```python
from build123d import *

# Parameters (mm, degrees)
SKETCH_W     = 53
SKETCH_H     = 50
PAD_DEPTH    = 2
SKETCH001_R  = 1.6
PAD001_DEPTH = 2
SKETCH002_R  = 1.6
PAD002_DEPTH = 2
SKETCH003_W  = 53
SKETCH003_H  = 4
PAD003_DEPTH = 6
POCKET_DEPTH = 50
FILLET_R     = 5


with BuildPart() as part:
    # Sketch → Pad (new body)
    with BuildSketch(Plane.YZ.offset(27)):
        Rectangle(SKETCH_W, SKETCH_H)
    extrude(amount=PAD_DEPTH)

    # Sketch001 (on Face4 of Pad) → Pad001 (join)
    with BuildSketch(Plane(origin=(27, -26.5, 0), x_dir=(0, 0, -1), z_dir=(0, -1, 0))):
        with BuildLine():
            Line((-32.5, 2), (32.5, 2))
            ThreePointArc((32.5, -8), (37.5, -3), (32.5, 2))
            Line((-32.5, -8), (32.5, -8))
            ThreePointArc((-32.5, 2), (-37.5, -3), (-32.5, -8))
        make_face()
        with Locations((-32.5, -3)):
            Circle(SKETCH001_R, mode=Mode.SUBTRACT)
        with Locations((32.5, -3)):
            Circle(SKETCH001_R, mode=Mode.SUBTRACT)
    extrude(amount=PAD001_DEPTH)

    # Sketch002 (on Face13 of Pad001) → Pad002 (join)
    with BuildSketch(Plane(origin=(27, 26.5, 0), x_dir=(0, 0, 1), z_dir=(0, 1, 0))):
        with BuildLine():
            Line((-32.5, 2), (32.5, 2))
            ThreePointArc((32.5, -8), (37.5, -3), (32.5, 2))
            Line((32.5, -8), (-32.5, -8))
            ThreePointArc((-32.5, 2), (-37.5, -3), (-32.5, -8))
        make_face()
        with Locations((-32.5, -3)):
            Circle(SKETCH002_R, mode=Mode.SUBTRACT)
        with Locations((32.5, -3)):
            Circle(SKETCH002_R, mode=Mode.SUBTRACT)
    extrude(amount=PAD002_DEPTH)

    # Sketch003 (on Face8 of Pad002) → Pad003 (join)
    with BuildSketch(Plane(origin=(27, 0, 0), x_dir=(0, 1, 0), z_dir=(-1, 0, 0))):
        with Locations((0, -15)):
            Rectangle(SKETCH003_W, SKETCH003_H)
        with Locations((0, 15)):
            Rectangle(SKETCH003_W, SKETCH003_H)
    extrude(amount=PAD003_DEPTH)

    # Sketch004 (on Face9 of Pad003) → Pocket (cut)
    with BuildSketch(Plane(origin=(27, 0, -17), x_dir=(0, 1, 0), z_dir=(0, 0, -1))):
        with BuildLine():
            ThreePointArc((-7, 0), (-7.942809, -0.390524), (-8.333333, -1.333333))
            Line((-8.333333, -2.666667), (-8.333333, -1.333333))
            ThreePointArc((-8.333333, -2.666667), (-7.942809, -3.609476), (-7, -4))
            Line((7, -4), (-7, -4))
            ThreePointArc((7, -4), (7.942809, -3.609476), (8.333333, -2.666667))
            Line((8.333333, -1.333333), (8.333333, -2.666667))
            ThreePointArc((8.333333, -1.333333), (7.942809, -0.390524), (7, 0))
            Line((-7, 0), (7, 0))
        make_face()
    extrude(amount=-POCKET_DEPTH, mode=Mode.SUBTRACT)

    # Fillet
    fillet_edges = [part.edges().sort_by_distance(p)[0] for p in [
        (27, 26.5, 0),
        (27, -26.5, 0),
        (27, 26.5, 21),
        (27, -26.5, 21),
        (27, -26.5, -21),
        (27, 26.5, -21),
    ]]
    fillet(fillet_edges, radius=FILLET_R)


solid = part.part
```
Design review of the part built by this model. Coordinates are the model's own, in mm. A direction names the side the tool comes from. Round coordinates to 2 decimals unless told otherwise and drop trailing zeros. Write each loop counter-clockwise with the first axis right and the second up, starting at its lowest first coordinate (ties: lowest second). Pieces come first, ordered by that corner, then holes.
Item 1: For faces 4 (the flat face through (21, 0, 15)), 5 (the cylindrical face through (25.57, -25, 21.06)), 6 (the flat face through (23, 0, 15)), list the 3-axis set-ups (+Z, -Z, +X, -X, +Y, -Y) from which the entire face can be reached by the end or side of a thin tool; tool diameter is ignored.
Item 2: The part is to be moulded in two halves that separate along Y. For faces 1 (the flat face through (28, 0, -25)), 2 (the flat face through (24, 28.5, 1)), 3 (the cylindrical face through (24.1, -27.5, 37.5)), say which applies: +Y half, -Y half, draft (parallel to the pull), parting line (faces both ways), or undercut.
Item 3: We need section A-A on y = 3.5. Write out the cut boundary in (x, z).
Item 4: We need section B-B on z = 16. Write out the cut boundary in (x, y), and give its area (3 significant figures).
Item 5: For probe 1 along X at (y, z) = (-27.6, -32.5); probe 2 along Y at (x, z) = (21.5, -7); probe 3 along Z at (x, y) = (22, 1.5), list the stretches that pass through material, from the lowest coordinate up.
Item 6: We need section C-C on z = -2.5. Write out the cut boundary in (x, y), and give its area (3 significant figures).
Item 7: Clearance check with flat-ended pins moving along their axes: pin 1 Ø4 at (y, z) = (2, -18.5) entering from -X; pin 2 Ø3 at (x, y) = (22, 0.5) entering from +Z; pin 3 Ø3 at (x, y) = (23.5, -12.5) entering from -Z. State where each tip first meets the part, or that it passes through.
Item 8: We need section D-D on y = 22.5. Write out the cut boundary in (x, z), and give its area (3 significant figures).
Returned:
1. face 4: +Z, -Z, -X
1. face 5: +Z, -X
1. face 6: +Z, -Z
2. face 1: undercut
2. face 2: +Y half
2. face 3: draft
3. outline: (21, -17) - (23, -17) - (23, -13) - (21, -13) - close; (21, 13) - (23, 13) - (23, 17) - (21, 17) - close; (27, -25) - (29, -25) - (29, 25) - (27, 25) - close
4. outline: (19, -28.5) - (29, -28.5) - (29, 28.5) - (19, 28.5) - (19, 26.5) - (21, 26.5) - (21, -26.5) - (19, -26.5) - close; hole (23, -7) arc R1.33 ccw to (24.33, -8.33) - (25.67, -8.33) arc R1.33 ccw to (27, -7) - (27, 7) arc R1.33 ccw to (25.67, 8.33) - (24.33, 8.33) arc R1.33 ccw to (23, 7) - close
4. area: 399 mm2
5. probe 1: x = 19 to 22.4, 25.6 to 29
5. probe 2: y = -28.5 to -26.5, 26.5 to 28.5
5. probe 3: z = -17 to -13, 13 to 17
6. outline: (19, -28.5) - (29, -28.5) - (29, 28.5) - (19, 28.5) - (19, 26.5) - (22, 26.5) arc R5 cw to (27, 21.5) - (27, -21.5) arc R5 cw to (22, -26.5) - (19, -26.5) - close
6. area: 157 mm2
7. pin 1: stops at x = 21
7. pin 2: stops at z = 17
7. pin 3: stops at z = -17
8. outline: (21, -17) - (26.9, -17) - (26.9, -25) - (29, -25) - (29, 25) - (26.9, 25) - (26.9, 17) - (21, 17) - (21, 13) - (26.9, 13) - (26.9, -13) - (21, -13) - close
8. area: 152 mm2
